```python
from build123d import *

# Parameters (mm, degrees)
SKETCH4_R           = 1
BOSS_EXTRUDE1_DEPTH = 3


with BuildPart() as part:
    # Sketch4 → Boss-Extrude1 (new body)
    with BuildSketch(Plane(origin=(454.145082272, -538.33265317, 0), x_dir=(0.7643426316132825, 0.6448103143549132, 0), z_dir=(0.6448103143549132, -0.7643426316132826, 0))):
        Polygon((554.951991089, 0), (554.951991089, 12), (546.701991089, 12), (546.701991089, 0), (550.951991089, 0), (550.951991089, -9), (554.951991089, -9), align=None)
        with Locations((552.951991089, 6)):
            Circle(SKETCH4_R, mode=Mode.SUBTRACT)
    extrude(amount=BOSS_EXTRUDE1_DEPTH)


solid = part.part
```
Part model, mm, in its own coordinate system. A direction names the side the tool comes from. Round coordinates to 2 decimals unless told otherwise and drop trailing zeros. Write each loop counter-clockwise with the first axis right and the second up, starting at its lowest first coordinate (ties: lowest second). Pieces come first, ordered by that corner, then holes. Notation, with made-up numbers: (36, 26.5) -> (47, 26.5) arc R21 cw to (47, 55.5) -> close; hole circle Ø6 at (-27.75, 86). An arc over 180 degrees is marked (long way). Return JSON: item names as keys, results as strings. Group by question number.
Q1. Saw through at A-A on z = 8.5. Write the cut outline in (x, y), plus the area to 4 significant figures.
Q2. Which spindle directions (+Z, -Z, +X, -X, +Y, -Y) get a long thin tool onto all of the face, cutting with end or side? Do faces 4 (the flat face through (875.82, -182.6, 3.98)), 5 (the flat face through (875, -186, 0)). Say none if no direction does.
Q3. Mould opens along Z. For faces 1 (the cylindrical face through (877.18, -183.389, 6.676)), 2 (the flat face through (876, -184, 12)), 3 (the flat face through (872.966, -186.944, 6.084)) say: pulls with the +Z half, pulls with the -Z half, needs draft (parallel to the pull), parting line crosses it, or undercut.
Q4. Pin check, flat tips, straight feed: pin 1 (1.5 mm diameter, centred on x = 879, z = -6.5, fed in from -Y); pin 2 (1 mm diameter, centred on y = -182.5, z = 9, fed in from -X); pin 3 (2 mm diameter, centred on x = 876.5, z = 9, fed in from -Y). Stop position of each tip, or through.
Q5. Saw through at C-C on y = -186.5. Write the cut outline in (x, z).
Q6. Saw through at B-B on x = 875.75. Write the cut outline in (y, z).
Q7. Probe L1, parallel to Z at x = 874.75, y = -184.75; L2, parallel to Z at x = 876.75, y = -182.5; L3, parallel to X at y = -186.25, z = 5. List the from-to ranges inside material, lowest first. Write a range as [from, to].
Answer:
{
 "1": {"outline": "(872.01, -185.81) -> (873.95, -188.11) -> (880.25, -182.79) -> (878.32, -180.49) -> close", "area": "24.75 mm2"},
 "2": {"face 4": "+Z, -Z, -X, +Y", "face 5": "-Z, -X, -Y"},
 "3": {"face 1": "undercut", "face 2": "pulls with the +Z half", "face 3": "needs draft"},
 "4": {"pin 1": "y = -184.48", "pin 2": "x = 875.35", "pin 3": "y = -186.8"},
 "5": {"outline": "(872.59, 0) -> (875.85, 0) -> (875.85, 12) -> (872.59, 12) -> close"},
 "6": {"outline": "(-186.59, 0) -> (-183.65, 0) -> (-183.65, -9) -> (-182.66, -9) -> (-182.66, 12) -> (-186.59, 12) -> close"},
 "7": {"L1": "[0, 12]", "L2": "[-9, 5.13], [6.87, 12]", "L3": "[872.38, 876.15]"}
}
